from build123d import *

# Parameters (mm, degrees)
CROQUIS2_R              = 1.75
SALIENTE_EXTRUIR1_DEPTH = 2


with BuildPart() as part:
    # Croquis2 → Saliente-Extruir1 (new body)
    with BuildSketch(Plane(origin=(0, 0, 0), x_dir=(0, 0, -1), z_dir=(1, 0, 0))):
        with BuildLine():
            ThreePointArc((-1624.025321873, 121.730654261), (-1586.485988342, -14.209738678), (-1539.232552396, -147.086014911))
            ThreePointArc((-1539.232552396, -147.086014911), (-1528.736264964, -158.30256709), (-1513.411789801, -159.371937759))
            ThreePointArc((-1513.411789801, -159.371937759), (-1405.508639065, -116.120173058), (-1305.452205903, -56.938121124))
            ThreePointArc((-1305.452205903, -56.938121124), (-1296.824738042, -43.452916514), (-1300.208231124, -27.805682905))
            ThreePointArc((-1300.208231124, -27.805682905), (-1377.246544078, 72.245539551), (-1464.284458168, 163.730785841))
            ThreePointArc((-1464.284458168, 163.730785841), (-1471.327397008, 168.136856279), (-1479.527832165, 169.467009446))
            ThreePointArc((-1479.527832165, 169.467009446), (-1545.52768268, 162.44811464), (-1609.97790425, 146.592071884))
            ThreePointArc((-1609.97790425, 146.592071884), (-1621.877582945, 136.916426614), (-1624.025321873, 121.730654261))
        make_face()
        with Locations((-1581.717582688, -12.705641768)):
            Circle(CROQUIS2_R, mode=Mode.SUBTRACT)
        with Locations((-1526.587976686, -153.787607791)):
            Circle(CROQUIS2_R, mode=Mode.SUBTRACT)
        with Locations((-1617.52441717, 134.456762464)):
            Circle(CROQUIS2_R, mode=Mode.SUBTRACT)
        with Locations((-1407.717991662, -111.634778861)):
            Circle(CROQUIS2_R, mode=Mode.SUBTRACT)
        with Locations((-1301.74565066, -42.567129287)):
            Circle(CROQUIS2_R, mode=Mode.SUBTRACT)
        with Locations((-1381.043785842, 68.992701562)):
            Circle(CROQUIS2_R, mode=Mode.SUBTRACT)
        with Locations((-1473.088384765, 163.457227863)):
            Circle(CROQUIS2_R, mode=Mode.SUBTRACT)
    extrude(amount=SALIENTE_EXTRUIR1_DEPTH)


solid = part.part
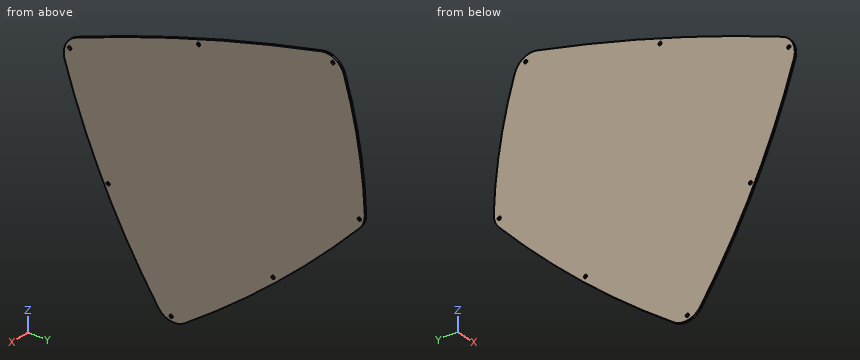
Work out the finished part from the listing and answer in its coordinate system (mm). Round coordinates to 2 decimals unless told otherwise and drop trailing zeros. Order: outer loops, then holes, each group sorted by start corner. A loop starts at its lowest first (then second) coordinate and runs counter-clockwise, first axis right, second up. Notation, with made-up numbers: M -16,85 L 17,85 A15 ccw 17,95 Z; hole C 81.5,33.5 d10. An arc over 180 degrees is marked long. Put each result on its own line as item: value. Start each with the question number.
Q1. A flat-ended cylindrical pin translates along its axis: pin 1 (1 mm diameter, centred on x = 1.5, z = 1410.5, fed in from +Y). Find the tip coordinate at first contact, or state that the pin passes through.
Q2. Section B-B, the plane z = 1495.5 is taken. Write down the section's boundary in (x, y), and give its area (3 significant figures).
Q3. Section C-C, the plane y = 86 is taken. Write down the section's boundary in (x, z).
Q4. Straight lines are drawn through the part: L1, parallel to Y at x = 1.65, z = 1313.5; L2, parallel to Y at x = 1.8, z = 1516.5; L3, parallel to Z at x = 0.9, y = 21.5. For each, find the intervals that lie inside material, in ascending order. Write a range as [from, to].
Q5. Section A-A, the plane x = 0.85 is taken. Write down the section's boundary in (y, z).
Findings below:
1. pin 1: stops at y = 110.02
2. outline: M 0,-153.49 L 2,-153.49 L 2,168.59 L 0,168.59 Z
2. area: 644 mm^2
3. outline: M 0,1389.21 L 2,1389.21 L 2,1615.18 L 0,1615.18 Z
4. L1: y = [-62.49, -8.93]
4. L2: y = [-160.09, 166.65]
4. L3: z = [1336.1, 1597.38]
5. outline: M -159.37,1513.41 A761 ccw -56.94,1305.45 A21 ccw -27.81,1300.21 A1211 ccw 163.73,1464.28 A21 ccw 169.47,1479.53 A491 ccw 146.59,1609.98 A21 ccw 121.73,1624.03 A1952.6 ccw -147.09,1539.23 A21 ccw Z; hole C -153.79,1526.59 d3.5; hole C -111.63,1407.72 d3.5; hole C -42.57,1301.75 d3.5; hole C -12.71,1581.72 d3.5; hole C 68.99,1381.04 d3.5; hole C 134.46,1617.52 d3.5; hole C 163.46,1473.09 d3.5
